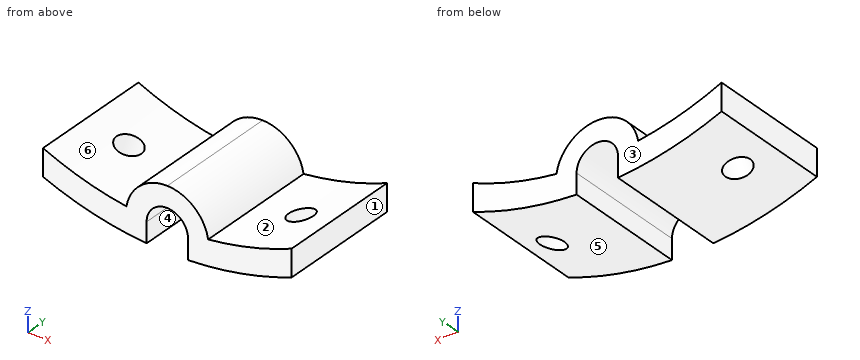
```python
from build123d import *

# Parameters (mm, degrees)
BOSS_EXTRU_1_DEPTH             = 15
D_GAGEMENT_M41_D               = 3.1
D_GAGEMENT_M41_DEPTH           = 30
D_GAGEMENT_M41_TIP             = 0.931333959
D_GAGEMENT_M41_ON_FACE_2_D     = 3.1
D_GAGEMENT_M41_ON_FACE_2_DEPTH = 30
D_GAGEMENT_M41_ON_FACE_2_TIP   = 0.931333959


with BuildPart() as part:
    # Esquisse1 → Boss.-Extru.1 (new body)
    with BuildSketch(Plane(origin=(0, 0, 0), x_dir=(1, 0, 0), z_dir=(0, 1, 0))):
        with BuildLine():
            Line((-2.5, 38.5), (-2.5, 40.923709509))
            ThreePointArc((-2.5, 40.923709509), (-8.858633339, 40.031545253), (-15, 38.157568057))
            Line((-15, 38.157568057), (-15, 34.9141805))
            ThreePointArc((-15, 34.9141805), (-10.061424249, 36.64379541), (-4.93206398, 37.678571429))
            ThreePointArc((-4.93206398, 37.678571429), (-3.232093528, 34.685085659), (0, 33.5))
            ThreePointArc((0, 33.5), (3.232093528, 34.685085659), (4.93206398, 37.678571429))
            ThreePointArc((4.93206398, 37.678571429), (10.061424249, 36.64379541), (15, 34.9141805))
            Line((15, 34.9141805), (15, 38.157568057))
            ThreePointArc((15, 38.157568057), (8.858633339, 40.031545253), (2.5, 40.923709509))
            Line((2.5, 40.923709509), (2.5, 38.5))
            ThreePointArc((2.5, 38.5), (0, 36), (-2.5, 38.5))
        make_face()
    extrude(amount=BOSS_EXTRU_1_DEPTH)

    # Dégagement M41
    with Locations(Plane(origin=(-11.210356129, 7.5, -39.437645917), x_dir=(-0.961893803, 0, 0.27342332), z_dir=(-0.27342332, 0, -0.961893803))):
        with Locations((0, 0)):
            Hole(D_GAGEMENT_M41_D / 2, depth=D_GAGEMENT_M41_DEPTH)
            with Locations((0, 0, -(D_GAGEMENT_M41_DEPTH + D_GAGEMENT_M41_TIP / 2))):  # 118° drill point
                Cone(0, D_GAGEMENT_M41_D / 2, D_GAGEMENT_M41_TIP, mode=Mode.SUBTRACT)

    # Dégagement M41 on face 2
    with Locations(Plane(origin=(11.210356129, 7.5, -39.437645917), x_dir=(-0.961893902, 0, -0.273422972), z_dir=(0.273422972, 0, -0.961893902))):
        with Locations((0, 0)):
            Hole(D_GAGEMENT_M41_ON_FACE_2_D / 2, depth=D_GAGEMENT_M41_ON_FACE_2_DEPTH)
            with Locations((0, 0, -(D_GAGEMENT_M41_ON_FACE_2_DEPTH + D_GAGEMENT_M41_ON_FACE_2_TIP / 2))):  # 118° drill point
                Cone(0, D_GAGEMENT_M41_ON_FACE_2_D / 2, D_GAGEMENT_M41_ON_FACE_2_TIP, mode=Mode.SUBTRACT)


solid = part.part
```
Part model, mm, in its own coordinate system. Face numbers are marked on the shaded views. A direction names the side the tool comes from. Round coordinates to 2 decimals unless told otherwise and drop trailing zeros. Loops run counter-clockwise (first coordinate to the right, second up) from the corner with the lowest first, then second, coordinate; pieces in that order, holes last. Notation, with made-up numbers: (-18, 25.5) -> (-14, 25.5) arc R20 ccw to (-14, 31.5) -> close; hole circle Ø11 at (-6, -2.5). An arc over 180 degrees is marked (long way). Use one line per item in the form item = value. Start each with the question number.
Item 1: Band-saw the part on C-C (x = -8). List the corners of the cut face in (y, z), plus the area to 3 significant figures.
Item 2: Tool access for the marked faces 4, 5 and 6: list every direction of +Z, -Z, +X, -X, +Y, -Y with a clear straight run to the whole face (end or side of a thin tool).
Item 3: Two-plate mould, pull along X, no slides. Class the marked faces 1, 2 and 3: released by +X, released by -X, zero draft, split by the parting line, or undercut.
Item 4: Band-saw the part on D-D (x = 2). List the corners of the cut face in (y, z).
Item 5: Drop a flat-ended pin along its axis: pin 1 Ø5 at (x, y) = (0.5, 10.5) entering from +Z. Give the stop position or say it passes through.
Item 6: Drill centre lines: line 1 along X through (y, z) = (2.5, -34.25); line 2 along Z through (x, y) = (1, 5); line 3 along Z through (x, y) = (4, 10.25). Where is each one in solid material? Low to high.
Item 7: Band-saw the part on B-B (y = 10). List the corners of the cut face in (x, z), plus the area to 3 significant figures.
Item 8: Band-saw the part on A-A (z = -35.5). List the corners of the cut face in (x, y).
Data:
q1.outline = (0, -40.21) -> (15, -40.21) -> (15, -37.15) -> (0, -37.15) -> close
q1.area = 46.0 mm^2
q2.face_4 = -Z, +Y, -Y
q2.face_5 = -Z, +X, +Y, -Y
q2.face_6 = +Z, +Y, -Y
q3.face_1 = released by +X
q3.face_2 = undercut
q3.face_3 = zero draft
q4.outline = (0, -37) -> (15, -37) -> (15, -33.92) -> (0, -33.92) -> close
q5.pin_1 = -33.5
q6.line_1 = -2.63 to 2.63
q6.line_2 = -36.21 to -33.6
q6.line_3 = -40.8 to -35.5
q7.outline = (-15, -38.16) arc R41 ccw to (-2.5, -40.92) -> (-2.5, -38.5) arc R2.5 cw to (2.5, -38.5) -> (2.5, -40.92) arc R41 ccw to (15, -38.16) -> (15, -34.91) arc R38 cw to (4.93, -37.68) arc R5 ccw to (-4.93, -37.68) arc R38 cw to (-15, -34.91) -> close
q7.area = 103 mm^2
q8.outline = (-15, 0) -> (-13.56, 0) -> (-13.56, 15) -> (-15, 15) -> close; (-4, 0) -> (4, 0) -> (4, 15) -> (-4, 15) -> close; (13.56, 0) -> (15, 0) -> (15, 15) -> (13.56, 15) -> close
